Geometry: see drawing. Coordinates: mm, zero at the bounding-box minimum. A direction names the side the tool comes from. Coordinates: 2 decimals unless noted, no trailing zeros. Loops run counter-clockwise (first coordinate to the right, second up) from the corner with the lowest first, then second, coordinate; pieces in that order, holes last.
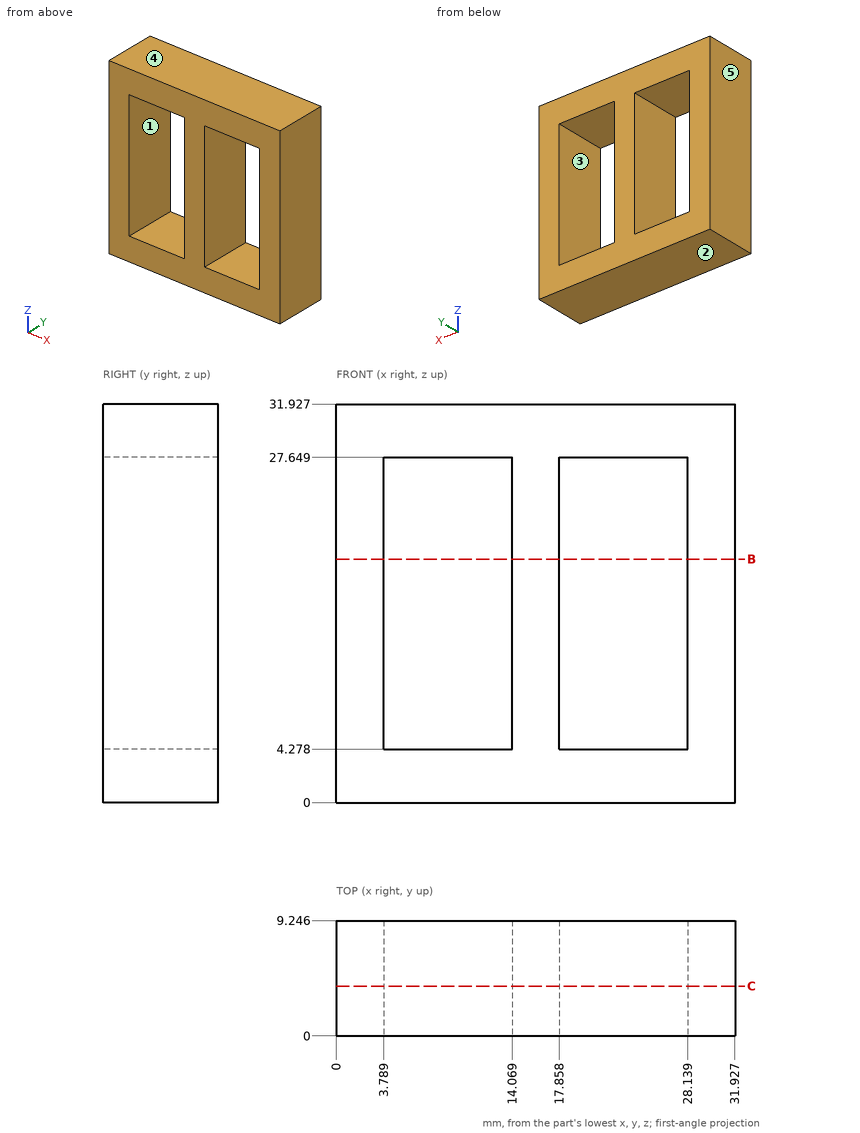
Item 1: Section query B-B (z = 19.5). Output: boundary loops of the cut face in (x, y) (1 decimal).
Result:
outline: (0, 0) - (3.8, 0) - (3.8, 9.2) - (0, 9.2) - close; (14.1, 0) - (17.9, 0) - (17.9, 9.2) - (14.1, 9.2) - close; (28.1, 0) - (31.9, 0) - (31.9, 9.2) - (28.1, 9.2) - close
Item 2: Reachability of the marked faces 1 and 2 from +Z, -Z, +X, -X, +Y, -Y: full face, straight path, thin tool, end or side. Return the list, or none.
Result:
face 1: +Y, -Y
face 2: -Z, +X, -X, +Y, -Y
Item 3: Section query C-C (y = 4). Output: boundary loops of the cut face in (x, z).
Result:
outline: (0, 0) - (31.93, 0) - (31.93, 31.93) - (0, 31.93) - close; hole (3.79, 4.28) - (14.07, 4.28) - (14.07, 27.65) - (3.79, 27.65) - close; hole (17.86, 4.28) - (28.14, 4.28) - (28.14, 27.65) - (17.86, 27.65) - close
Item 4: Line query: L1, parallel to X at y = 6.25, z = 25; L2, parallel to Z at x = 8, y = 7. Output: solid intervals per line, ascending.
Result:
L1: x = 0 to 3.79, 14.07 to 17.86, 28.14 to 31.93
L2: z = 0 to 4.28, 27.65 to 31.93
Item 5: Mould query, pull axis Z, two halves, no side actions, for the marked faces 3, 4 and 5. Classes: +Z half, -Z half, draft (parallel to the pull), parting line (faces both ways), or undercut.
Result:
face 3: undercut
face 4: +Z half
face 5: draft
Item 6: Contact query for a flat-ended pin moving along its axis: P1, Ø3, axis at y = 5, z = 13, coming from the -X side. Output: stop coordinate, or through.
Result:
P1: stops at x = 0
